Input: part model. Units: mm. Frame: model coordinates. Coordinates: 2 decimals unless noted, no trailing zeros.
from build123d import *

# Parameters (mm, degrees)
F0_R     = 3
F0_R_2   = 2.5
F1_DEPTH = 565


with BuildPart() as f1:
    # F0 (on Front) → F1 (new body)
    with BuildSketch(Plane.XZ):
        with BuildLine():
            Line((-4.5, 15), (-14, 15))
            ThreePointArc((-14, 15), (-14.707107, 14.707107), (-15, 14))
            Line((-15, 14), (-15, 4.5))
            ThreePointArc((-15, 4.5), (-14.912132, 4.287868), (-14.7, 4.2))
            Line((-14.7, 4.2), (-14.5, 4.2))
            ThreePointArc((-14.5, 4.2), (-14.146447, 4.053553), (-14, 3.7))
            Line((-14, 3.7), (-14, 3.55))
            ThreePointArc((-14, 3.55), (-13.912132, 3.337868), (-13.7, 3.25))
            Line((-13.7, 3.25), (-12.5, 3.25))
            Line((-12.5, 3.25), (-12.5, 5.25))
            Line((-12.5, 5.25), (-8.004644, 5.25))
            ThreePointArc((-8.004644, 5.25), (-7.629545, 5.176985), (-7.309222, 4.968602))
            Line((-7.309222, 4.968602), (-4.804579, 2.544753))
            ThreePointArc((-4.804579, 2.544753), (-4.579288, 2.216394), (-4.5, 1.826151))
            Line((-4.5, 1.826151), (-4.5, -1.826151))
            ThreePointArc((-4.5, -1.826151), (-4.579288, -2.216394), (-4.804579, -2.544753))
            Line((-4.804579, -2.544753), (-7.309222, -4.968602))
            ThreePointArc((-7.309222, -4.968602), (-7.629545, -5.176985), (-8.004644, -5.25))
            Line((-8.004644, -5.25), (-12.5, -5.25))
            Line((-12.5, -5.25), (-12.5, -3.25))
            Line((-12.5, -3.25), (-13.7, -3.25))
            ThreePointArc((-13.7, -3.25), (-13.912132, -3.337868), (-14, -3.55))
            Line((-14, -3.55), (-14, -3.7))
            ThreePointArc((-14, -3.7), (-14.146447, -4.053553), (-14.5, -4.2))
            Line((-14.5, -4.2), (-14.7, -4.2))
            ThreePointArc((-14.7, -4.2), (-14.912132, -4.287868), (-15, -4.5))
            Line((-15, -4.5), (-15, -14))
            ThreePointArc((-15, -14), (-14.707107, -14.707107), (-14, -15))
            Line((-14, -15), (-4.5, -15))
            ThreePointArc((-4.5, -15), (-4.287868, -14.912132), (-4.2, -14.7))
            Line((-4.2, -14.7), (-4.2, -14.5))
            ThreePointArc((-4.2, -14.5), (-4.053553, -14.146447), (-3.7, -14))
            Line((-3.7, -14), (-3.55, -14))
            ThreePointArc((-3.55, -14), (-3.337868, -13.912132), (-3.25, -13.7))
            Line((-3.25, -13.7), (-3.25, -12.5))
            Line((-3.25, -12.5), (-5.25, -12.5))
            Line((-5.25, -12.5), (-5.25, -8.004644))
            ThreePointArc((-5.25, -8.004644), (-5.176985, -7.629545), (-4.968602, -7.309222))
            Line((-4.968602, -7.309222), (-2.544753, -4.804579))
            ThreePointArc((-2.544753, -4.804579), (-2.216394, -4.579288), (-1.826151, -4.5))
            Line((-1.826151, -4.5), (1.826151, -4.5))
            ThreePointArc((1.826151, -4.5), (2.216394, -4.579288), (2.544753, -4.804579))
            Line((2.544753, -4.804579), (4.968602, -7.309222))
            ThreePointArc((4.968602, -7.309222), (5.176985, -7.629545), (5.25, -8.004644))
            Line((5.25, -8.004644), (5.25, -12.5))
            Line((5.25, -12.5), (3.25, -12.5))
            Line((3.25, -12.5), (3.25, -13.7))
            ThreePointArc((3.25, -13.7), (3.337868, -13.912132), (3.55, -14))
            Line((3.55, -14), (3.7, -14))
            ThreePointArc((3.7, -14), (4.053553, -14.146447), (4.2, -14.5))
            Line((4.2, -14.5), (4.2, -14.7))
            ThreePointArc((4.2, -14.7), (4.287868, -14.912132), (4.5, -15))
            Line((4.5, -15), (14, -15))
            ThreePointArc((14, -15), (14.707107, -14.707107), (15, -14))
            Line((15, -14), (15, -4.5))
            ThreePointArc((15, -4.5), (14.912132, -4.287868), (14.7, -4.2))
            Line((14.7, -4.2), (14.5, -4.2))
            ThreePointArc((14.5, -4.2), (14.146447, -4.053553), (14, -3.7))
            Line((14, -3.7), (14, -3.55))
            ThreePointArc((14, -3.55), (13.912132, -3.337868), (13.7, -3.25))
            Line((13.7, -3.25), (12.5, -3.25))
            Line((12.5, -3.25), (12.5, -5.25))
            Line((12.5, -5.25), (8.004644, -5.25))
            ThreePointArc((8.004644, -5.25), (7.629545, -5.176985), (7.309222, -4.968602))
            Line((7.309222, -4.968602), (4.804579, -2.544753))
            ThreePointArc((4.804579, -2.544753), (4.579288, -2.216394), (4.5, -1.826151))
            Line((4.5, -1.826151), (4.5, 1.826151))
            ThreePointArc((4.5, 1.826151), (4.579288, 2.216394), (4.804579, 2.544753))
            Line((4.804579, 2.544753), (7.309222, 4.968602))
            ThreePointArc((7.309222, 4.968602), (7.629545, 5.176985), (8.004644, 5.25))
            Line((8.004644, 5.25), (12.5, 5.25))
            Line((12.5, 5.25), (12.5, 3.25))
            Line((12.5, 3.25), (13.7, 3.25))
            ThreePointArc((13.7, 3.25), (13.912132, 3.337868), (14, 3.55))
            Line((14, 3.55), (14, 3.7))
            ThreePointArc((14, 3.7), (14.146447, 4.053553), (14.5, 4.2))
            Line((14.5, 4.2), (14.7, 4.2))
            ThreePointArc((14.7, 4.2), (14.912132, 4.287868), (15, 4.5))
            Line((15, 4.5), (15, 14))
            ThreePointArc((15, 14), (14.707107, 14.707107), (14, 15))
            Line((14, 15), (4.5, 15))
            ThreePointArc((4.5, 15), (4.287868, 14.912132), (4.2, 14.7))
            Line((4.2, 14.7), (4.2, 14.5))
            ThreePointArc((4.2, 14.5), (4.053553, 14.146447), (3.7, 14))
            Line((3.7, 14), (3.55, 14))
            ThreePointArc((3.55, 14), (3.337868, 13.912132), (3.25, 13.7))
            Line((3.25, 13.7), (3.25, 12.5))
            Line((3.25, 12.5), (5.25, 12.5))
            Line((5.25, 12.5), (5.25, 8.004644))
            ThreePointArc((5.25, 8.004644), (5.176985, 7.629545), (4.968602, 7.309222))
            Line((4.968602, 7.309222), (2.544753, 4.804579))
            ThreePointArc((2.544753, 4.804579), (2.216394, 4.579288), (1.826151, 4.5))
            Line((1.826151, 4.5), (-1.826151, 4.5))
            ThreePointArc((-1.826151, 4.5), (-2.216394, 4.579288), (-2.544753, 4.804579))
            Line((-2.544753, 4.804579), (-4.968602, 7.309222))
            ThreePointArc((-4.968602, 7.309222), (-5.176985, 7.629545), (-5.25, 8.004644))
            Line((-5.25, 8.004644), (-5.25, 12.5))
            Line((-5.25, 12.5), (-3.25, 12.5))
            Line((-3.25, 12.5), (-3.25, 13.7))
            ThreePointArc((-3.25, 13.7), (-3.337868, 13.912132), (-3.55, 14))
            Line((-3.55, 14), (-3.7, 14))
            ThreePointArc((-3.7, 14), (-4.053553, 14.146447), (-4.2, 14.5))
            Line((-4.2, 14.5), (-4.2, 14.7))
            ThreePointArc((-4.2, 14.7), (-4.287868, 14.912132), (-4.5, 15))
        make_face()
        with Locations((-10, -10)):
            Circle(F0_R, mode=Mode.SUBTRACT)
        with Locations((10, -10)):
            Circle(F0_R, mode=Mode.SUBTRACT)
        with Locations((-10, 10)):
            Circle(F0_R, mode=Mode.SUBTRACT)
        Circle(F0_R_2, mode=Mode.SUBTRACT)
        with Locations((10, 10)):
            Circle(F0_R, mode=Mode.SUBTRACT)
    extrude(amount=F1_DEPTH)


solid = f1.part
Item 1: Section query A-A, the plane y = -261. State how many separate pieces and enclosed holes the cut face has, then the cut area to 3 significant figures.
Item 2: Material intervals for line 1 (Z direction, x = -10.5, y = -221.5); line 2 (X direction, y = -438.5, z = 8.5); line 3 (Z direction, x = -8, y = -30.5), sorted ascending.
Item 3: Pin query (flat end, axial travel): pin 1 Ø5 at (y, z) = (-184, 0) entering from +X; pin 2 Ø3 at (x, z) = (11.5, -3.5) entering from +Y; pin 3 Ø4 at (x, y) = (-1, -319) entering from +Z (3 decimals). Return the tip coordinate at first contact, or that it passes through.
The answers:
1. separate pieces: 1
1. enclosed holes: 5
1. area: 395 mm2
2. line 1: z = -15 to -12.96, -7.04 to -5.25, 5.25 to 7.04, 12.96 to 15
2. line 2: x = -15 to -12.6, -7.4 to -5.25, 5.25 to 7.4, 12.6 to 15
2. line 3: z = -15 to -12.24, -7.76 to -5.25, 5.25 to 7.76, 12.24 to 15
3. pin 1: stops at x = 4.76
3. pin 2: stops at y = 0
3. pin 3: stops at z = 5.275
